For this review, take the finished solid that the model builds, in its own axes (mm). Coordinates: 2 decimals unless noted, no trailing zeros. Write each loop counter-clockwise with the first axis right and the second up, starting at its lowest first coordinate (ties: lowest second). Pieces come first, ordered by that corner, then holes. Notation, with made-up numbers: M 18,87 L 26,87 A16 cw 26,93 Z; hole C -23,76 d1. An arc over 180 degrees is marked long. One line per question, with ' | ' between items.
from build123d import *

# Parameters (mm, degrees)
BOSS_EXTRUDE1_DEPTH                       = 17.78
SKETCH3_R                                 = 3
CUT_EXTRUDE3_DEPTH                        = 6
CUT_EXTRUDE4_START                        = -6
SKETCH4_R                                 = 3
CUT_EXTRUDE4_DEPTH                        = 6
TAP_DRILL_FOR_M4X0_7_TAP1_D               = 3.3
TAP_DRILL_FOR_M4X0_7_TAP1_DEPTH           = 10
TAP_DRILL_FOR_M4X0_7_TAP1_TIP             = 0.991420021
TAP_DRILL_FOR_M4X0_7_TAP1_ON_FACE_2_D     = 3.3
TAP_DRILL_FOR_M4X0_7_TAP1_ON_FACE_2_DEPTH = 10
TAP_DRILL_FOR_M4X0_7_TAP1_ON_FACE_2_TIP   = 0.991420021


with BuildPart() as part:
    # Sketch1 → Boss-Extrude1 (new body)
    with BuildSketch(Plane(origin=(0, 0, 0), x_dir=(-0.044080076933776656, 0.9990280010177455, 0), z_dir=(0, 0, 1))):
        with BuildLine():
            Line((-5.997717637, -62.816664904), (-5.997717637, -63.551933441))
            Line((-5.997717637, -63.551933441), (-145.997717637, -63.551933441))
            Line((-145.997717637, -63.551933441), (-145.997717637, 73.188066556))
            Line((-145.997717637, 73.188066556), (-5.997717637, 73.188066556))
            Line((-5.997717637, 73.188066556), (-5.997717637, 72.452798018))
            ThreePointArc((-5.997717637, 72.452798018), (-64.367717636, 4.818066557), (-5.997717637, -62.816664904))
        make_face()
    extrude(amount=BOSS_EXTRUDE1_DEPTH)

    # Sketch3 → Cut-Extrude3 (cut)
    with BuildSketch(Plane(origin=(-73.116927829, -3.226135604, 0), x_dir=(0, 0, 1), z_dir=(-0.9990280010177455, -0.044080076933776635, 0))):
        with Locations(Location((8.89, -62.227710676, 0), (0, 0, 270))):
            Circle(SKETCH3_R)
    extrude(amount=-CUT_EXTRUDE3_DEPTH, mode=Mode.SUBTRACT)

    # Sketch4 → Cut-Extrude4 (cut)
    with BuildSketch(Plane(origin=(63.490161027, 2.801374115, 0), x_dir=(0, 0, -1), z_dir=(0.9990280010177455, 0.044080076933776635, 0)).offset(CUT_EXTRUDE4_START)):
        with Locations(Location((-8.89, -62.227710676, 0), (0, 0, 270))):
            Circle(SKETCH4_R)
    extrude(amount=CUT_EXTRUDE4_DEPTH, mode=Mode.SUBTRACT)

    # Tap Drill for M4x0.7 Tap1
    with Locations(Plane(origin=(-32.52956499, -147.575066179, 8.89), x_dir=(-0.999028001018, -0.044080076934, 0), z_dir=(0.044080076934, -0.999028001018, 0))):
        with Locations((0, 0)):
            Hole(TAP_DRILL_FOR_M4X0_7_TAP1_D / 2, depth=TAP_DRILL_FOR_M4X0_7_TAP1_DEPTH)
            with Locations((0, 0, -(TAP_DRILL_FOR_M4X0_7_TAP1_DEPTH + TAP_DRILL_FOR_M4X0_7_TAP1_TIP / 2))):  # 118° drill point
                Cone(0, TAP_DRILL_FOR_M4X0_7_TAP1_D / 2, TAP_DRILL_FOR_M4X0_7_TAP1_TIP, mode=Mode.SUBTRACT)

    # Tap Drill for M4x0.7 Tap1 on face 2
    with Locations(Plane(origin=(35.773979438, -144.561311319, 8.89), x_dir=(-0.999028004404, -0.044080000194, 0), z_dir=(0.044080000194, -0.999028004404, 0))):
        with Locations((0, 0)):
            Hole(TAP_DRILL_FOR_M4X0_7_TAP1_ON_FACE_2_D / 2, depth=TAP_DRILL_FOR_M4X0_7_TAP1_ON_FACE_2_DEPTH)
            with Locations((0, 0, -(TAP_DRILL_FOR_M4X0_7_TAP1_ON_FACE_2_DEPTH + TAP_DRILL_FOR_M4X0_7_TAP1_ON_FACE_2_TIP / 2))):  # 118° drill point
                Cone(0, TAP_DRILL_FOR_M4X0_7_TAP1_ON_FACE_2_D / 2, TAP_DRILL_FOR_M4X0_7_TAP1_ON_FACE_2_TIP, mode=Mode.SUBTRACT)


solid = part.part
1. Take a section at A-A on y = -49. State the section outline as (x, z) points.
Computed values:
outline: M -71.1,0 L -48.44,0 L -48.44,17.78 L -71.1,17.78 Z; M 38.46,0 L 65.78,0 L 65.78,17.78 L 38.46,17.78 Z
2. Take a section at C-C on y = -14.5. State the section outline as (x, z) points.
Computed values:
outline: M -72.62,0 L -70.87,0 L -70.87,17.78 L -72.62,17.78 Z; M 60.89,0 L 64.25,0 L 64.25,17.78 L 60.89,17.78 Z
3. Take a section at B-B on z = 15.5. State the section outline as (x, y) points, plus the area to 3 significant figures.
Computed values:
outline: M -72.85,-9.22 L -66.68,-149.08 L 69.93,-143.05 L 63.75,-3.19 L 63.02,-3.22 A68.37 cw -72.12,-9.19 Z | area: 13,200 mm2
4. Take a section at D-D on x = 26.5. State the section outline as (y, z) points, plus the area to 3 significant figures.
Computed values:
outline: M -144.97,0 L -56.9,0 L -56.9,17.78 L -144.97,17.78 Z | area: 1,570 mm2
5. Draft analysis for pull direction X (two halves, no side actions). For faces 1 (the flat face through (-2, -91, 17.78)), 2 (the cylindrical face through (-67.55, -62.27, 9.02)), 3 (the flat face through (2.578, -146.026, 8.766)), state which applies: pulls with the +X half, pulls with the -X half, needs draft (parallel to the pull), parting line crosses it, or undercut.
Computed values:
face 1: needs draft | face 2: undercut | face 3: pulls with the +X half
6. For line 1 along X through (y, z) = (-137.5, 8.75); line 2 along X through (y, z) = (-55, 16.25); line 3 along X through (y, z) = (-17, 8), list the stretches that pass through material, from the lowest coordinate up.
Computed values:
line 1: x = -67.19 to -34.37, -31.35 to 33.82, 37.11 to 69.68 | line 2: x = -70.83 to -39.9, 29.92 to 66.04 | line 3: x = -72.51 to -70.12, 60.14 to 64.36
7. Clearance check with flat-ended pins moving along their axes: P1, Ø8, axis at y = -19, z = 3, coming from the -X side; P2, Ø1, axis at x = -30.5, z = 14.5, coming from the +Y side; P3, Ø2, axis at x = -50, z = 6, coming from the -Y side; P4, Ø8, axis at x = -2.5, y = -57.5, coming from the +Z side. State where each tip first meets the part, or that it passes through.
Computed values:
P1: stops at x = -72.6 | P2: stops at y = -59.44 | P3: stops at y = -148.39 | P4: passes through
